For this review, take the finished solid that the model builds, in its own axes (mm). A direction names the side the tool comes from. Coordinates: 2 decimals unless noted, no trailing zeros. Loops run counter-clockwise (first coordinate to the right, second up) from the corner with the lowest first, then second, coordinate; pieces in that order, holes last. Notation, with made-up numbers: M -31.5,85.5 L -0.5,85.5 A8 cw -0.5,95.5 Z; hole C -5,88.5 d3. An arc over 180 degrees is marked long. Use one line per item in the form item = value.
Autodesk Inventor part; units mm, degrees
ref_plane "YZ Plane" through (0, 0, 0) normal (1, 0, 0) x (0, 1, 0)
ref_plane "XZ Plane" through (0, 0, 0) normal (0, 1, 0) x (-1, 0, 0)
ref_plane "XY Plane" through (0, 0, 0) normal (0, 0, 1) x (1, 0, 0)
sketch "Sketch1" plane through (0, 0, 0) normal (0, 0, 1) x (1, 0, 0)
  line L0 (0, 0) -> (50, 0) construction
  line L1 (50, 0) -> (50, 20) construction
  line L2 (50, 0.7657) -> (0, 0.7657) construction
  line L3 (0, 20) -> (0, 0) construction
  spline S0 degree 2 poles (17.0019, 5.3908) (17.0019, 3.0567) (11.2962, 0.5208) (6.4982, 0.5208) knots 0 0 0 1 2 2 2
  spline S1 degree 2 poles (6.4982, 0.5208) (5.3455, 0.5208) (1.4985, 0.7225) (0.2161, 0.8666) knots 0 0 0 1 2 2 2
  line L4 (0.2161, 0.8666) -> (0.2161, 3.1431)
  line L5 (0.2161, 3.1431) -> (0.4755, 3.1431)
  spline S2 degree 2 poles (0.4755, 3.1431) (1.4553, 2.9702) (4.3513, 2.5668) (5.8498, 2.5668) knots 0 0 0 1 2 2 2
  spline S3 degree 2 poles (5.8498, 2.5668) (8.0543, 2.5668) (10.6478, 3.0711) (11.2674, 3.5321) knots 0 0 0 1 2 2 2
  spline S4 degree 2 poles (11.2674, 3.5321) (11.9158, 4.0076) (12.276, 5.3908) (12.276, 6.2986) knots 0 0 0 1 2 2 2
  line L6 (12.276, 6.2986) -> (12.276, 16.6582)
  line L7 (12.276, 16.6582) -> (4.7548, 16.6582)
  line L8 (4.7548, 16.6582) -> (4.7548, 18.5457)
  line L9 (4.7548, 18.5457) -> (17.0019, 18.5457)
  line L10 (17.0019, 18.5457) -> (17.0019, 5.3908)
  line L11 (45.2569, 16.4421) -> (28.7016, 16.4421)
  line L12 (28.7016, 16.4421) -> (28.7016, 11.428)
  line L13 (28.7016, 11.428) -> (44.5653, 11.428)
  line L14 (44.5653, 11.428) -> (44.5653, 9.3243)
  line L15 (44.5653, 9.3243) -> (28.7016, 9.3243)
  line L16 (28.7016, 9.3243) -> (28.7016, 0.7657)
  line L17 (28.7016, 0.7657) -> (23.9756, 0.7657)
  line L18 (23.9756, 0.7657) -> (23.9756, 18.5457)
  line L19 (23.9756, 18.5457) -> (45.2569, 18.5457)
  line L20 (45.2569, 18.5457) -> (45.2569, 16.4421)
  dimension "d0" = 50
  dimension "d1" = 20
extrude "Extrusion1" add sketch "Sketch1" along normal blind 10
sketch "Sketch2" plane through (0, 0, 0) normal (1, 0, 0) x (0, 1, 0)
  point P0 (0, 0)
sketch "Sketch3" plane through (0, 0, 0) normal (0, 0, 1) x (1, 0, 0)
  line L0 (0, 0) -> (50, 0)
  line L1 (50, 0) -> (50, 0.8967)
  line L2 (50, 0.8967) -> (0, 0.8967)
  line L3 (0, 0.8967) -> (0, 0)
  dimension "d4" = 50
extrude "Extrusion2" add sketch "Sketch3" along normal blind 10
properties part number "jf_inits"
1. Consider section B-B on x = 39.5. Write out the cut boundary in (y, z).
Computed values:
outline = M 0,0 L 0.9,0 L 0.9,10 L 0,10 Z; M 9.32,0 L 11.43,0 L 11.43,10 L 9.32,10 Z; M 16.44,0 L 18.55,0 L 18.55,10 L 16.44,10 Z
2. Draft analysis for pull direction X (two halves, no side actions). For faces 6 (the face through (9, 16.658, 5)), 7 (the face through (44.565, 10, 5)), 8 (the face through (18, 0.897, 5)), state which applies: +X half, -X half, draft (parallel to the pull), parting line (faces both ways), or undercut.
Computed values:
face_6 = draft
face_7 = +X half
face_8 = undercut
3. For pin 1 Ø5 at (y, z) = (10.5, 7.5) entering from -X; pin 2 Ø2.5 at (y, z) = (10.5, 5.5) entering from +X; pin 3 Ø3 at (y, z) = (13.5, 3.5) entering from +X, all flat-tipped, find the tip position at first contact; note any pin that passes through.
Computed values:
pin_1 = 12.28
pin_2 = 44.57
pin_3 = 28.7
4. Consider section C-C on x = 20. Write out the cut boundary in (y, z).
Computed values:
outline = M 0,0 L 0.9,0 L 0.9,10 L 0,10 Z
5. Consider section A-A on y = 8.75. Write out the cut boundary in (x, z), plus the area to 3 significant figures.
Computed values:
outline = M 12.28,0 L 17,0 L 17,10 L 12.28,10 Z; M 23.98,0 L 28.7,0 L 28.7,10 L 23.98,10 Z
area = 94.5 mm2
6. Tool access review of faces 1 (the face through (28.702, 14, 5)), 2 (the face through (45.257, 18, 5)), 3 (the face through (12.276, 11, 5)), 4 (the face through (23.976, 10, 5)), 5 (the face through (4.755, 18, 5)): name each direction out of +Z, -Z, +X, -X, +Y, -Y from which nothing blocks a thin tool from reaching the whole face with its end or side.
Computed values:
face_1 = +Z, -Z, +X
face_2 = +Z, -Z, +X, +Y
face_3 = +Z, -Z, -X
face_4 = +Z, -Z, +Y
face_5 = +Z, -Z, -X, +Y
7. Wall thickness on line 1 along Y through (x, z) = (42.5, 1.5); line 2 along Y through (x, z) = (15.5, 2.5); line 3 along X through (y, z) = (6, 4.25): over which ranges is each line inside the solid? List them lowest first. Write a range as from..to.
Computed values:
line_1 = 0..0.9, 9.32..11.43, 16.44..18.55
line_2 = 0..0.9, 2.56..18.55
line_3 = 12.27..17, 23.98..28.7
